Could you check a few things on this model? Use its own coordinates, in mm. A direction names the side the tool comes from. Give positions to 0.01 mm unless a question says otherwise; leave off trailing zeros. Loops run counter-clockwise (first coordinate to the right, second up) from the corner with the lowest first, then second, coordinate; pieces in that order, holes last. Notation, with made-up numbers: (75, 6.25) - (99, 6.25) arc R21 ccw to (99, 13.25) - close; hole circle Ø10 at (-34, -33.75). An arc over 180 degrees is marked (long way). Answer in a Markdown table with one row per item. Add a question column.
```python
from build123d import *

# Parameters (mm, degrees)
F1_DEPTH = 22
F3_DEPTH = 45.181


with BuildPart() as f1:
    # F0 (on Front) → F1 (new body, symmetric)
    with BuildSketch(Plane.XZ):
        Polygon((0, 45.18), (0, 0), (1.9, 0), (1.9, 43.28), (21.2, 43.28), (21.2, 45.18), align=None)
    extrude(amount=F1_DEPTH, both=True)

    # F2 (on face) → F3 (cut, through all)
    with BuildSketch(Plane.XY.offset(45.18)):
        with BuildLine():
            ThreePointArc((11.6, -12.5), (8.1, -16), (11.6, -19.5))
            Line((11.6, -19.5), (14.6, -19.5))
            ThreePointArc((14.6, -19.5), (18.1, -16), (14.6, -12.5))
            Line((14.6, -12.5), (11.6, -12.5))
        make_face()
        with BuildLine():
            ThreePointArc((11.6, 19.5), (8.1, 16), (11.6, 12.5))
            Line((11.6, 12.5), (14.6, 12.5))
            ThreePointArc((14.6, 12.5), (18.1, 16), (14.6, 19.5))
            Line((14.6, 19.5), (11.6, 19.5))
        make_face()
        with BuildLine():
            ThreePointArc((14.9, 7.05), (12.85, 9.1), (10.8, 7.05))
            Line((10.8, 7.05), (10.8, 3.434749))
            ThreePointArc((10.8, 3.434749), (12.85, 4), (14.9, 3.434749))
            Line((14.9, 3.434749), (14.9, 7.05))
        make_face()
        with BuildLine():
            ThreePointArc((14.9, 3.434749), (12.85, 4), (10.8, 3.434749))
            ThreePointArc((10.8, 3.434749), (8.85, 0), (10.8, -3.434749))
            ThreePointArc((10.8, -3.434749), (12.85, -4), (14.9, -3.434749))
            ThreePointArc((14.9, -3.434749), (16.328505, -1.974842), (16.85, 0))
            ThreePointArc((16.85, 0), (16.328505, 1.974842), (14.9, 3.434749))
        make_face()
        with BuildLine():
            ThreePointArc((14.9, -3.434749), (12.85, -4), (10.8, -3.434749))
            Line((10.8, -3.434749), (10.8, -7.05))
            ThreePointArc((10.8, -7.05), (12.85, -9.1), (14.9, -7.05))
            Line((14.9, -7.05), (14.9, -3.434749))
        make_face()
    extrude(amount=-F3_DEPTH, mode=Mode.SUBTRACT)


solid = f1.part
```
(1) Please list where these lines run through material, in increasing order: line 1 (X direction, y = 18, z = 30.5); line 2 (Z direction, x = 19.25, y = 7.5).
(2) I want a section at B-B on x = 12.85. Please give me the cut outline in (y, z), then the cut area to 3 significant figures.
(3) For pin 1 Ø6 at (x, y) = (9.5, -1.5) entering from -Z; pin 2 Ø8 at (y, z) = (-16, 33.5) entering from +X, each with a flat end and sliding along its axis, tell me the tip position at first contact or that it passes through.
(4) I want a section at A-A on y = -6.5. Please give me the cut outline in (x, z), then the cut area to 3 significant figures.
(5) I want a section at D-D on y = 16. Please give me the cut outline in (x, z).
(6) I want a section at C-C on y = 10.5. Please give me the cut outline in (x, z), then the cut area to 3 significant figures.
(7) On a 3-axis mill with a long thin cutter (end or side, diameter ignored), from which of +Z, -Z, +X, -X, +Y, -Y can I reach the whole of each face in a straight line? I mean faces 1 (the flat face through (8, 0, 45.18)), 2 (the flat face through (13, 19.5, 44)), 3 (the flat face through (1.9, 0, 21)). Say none if no direction works.
(8) We'd pull the mould along X, two halves only. Please class faces 4 (the flat face through (0, 0, 23)), 5 (the flat face through (13, -12.5, 44)), 6 (the flat face through (21.2, 0, 44)): pulls with the +X half, pulls with the -X half, needs draft (parallel to the pull), parting line crosses it, or undercut.
Reported:
| question | item | result |
|---|---|---|
| 1 | line 1 | 0 to 1.9 |
| 1 | line 2 | 43.28 to 45.18 |
| 2 | outline | (-22, 43.28) - (-19.5, 43.28) - (-19.5, 45.18) - (-22, 45.18) - close; (-12.5, 43.28) - (-9.1, 43.28) - (-9.1, 45.18) - (-12.5, 45.18) - close; (9.1, 43.28) - (12.5, 43.28) - (12.5, 45.18) - (9.1, 45.18) - close; (19.5, 43.28) - (22, 43.28) - (22, 45.18) - (19.5, 45.18) - close |
| 2 | area | 22.4 mm² |
| 3 | pin 1 | z = 43.28 |
| 3 | pin 2 | x = 1.9 |
| 4 | outline | (0, 0) - (1.9, 0) - (1.9, 43.28) - (10.8, 43.28) - (10.8, 45.18) - (0, 45.18) - close; (14.9, 43.28) - (21.2, 43.28) - (21.2, 45.18) - (14.9, 45.18) - close |
| 4 | area | 115 mm² |
| 5 | outline | (0, 0) - (1.9, 0) - (1.9, 43.28) - (8.1, 43.28) - (8.1, 45.18) - (0, 45.18) - close; (18.1, 43.28) - (21.2, 43.28) - (21.2, 45.18) - (18.1, 45.18) - close |
| 6 | outline | (0, 0) - (1.9, 0) - (1.9, 43.28) - (21.2, 43.28) - (21.2, 45.18) - (0, 45.18) - close |
| 6 | area | 123 mm² |
| 7 | face 1 | +Z, +X, -X, +Y, -Y |
| 7 | face 2 | +Z, -Z |
| 7 | face 3 | -Z, +X, +Y, -Y |
| 8 | face 4 | pulls with the -X half |
| 8 | face 5 | undercut |
| 8 | face 6 | pulls with the +X half |
